Answer from the drawing. Dimensions are ordinates in mm from the lowest x, y and z of the part. A direction names the side the tool comes from. Give positions to 0.01 mm unless a question says otherwise; leave off trailing zeros. Loops run counter-clockwise (first coordinate to the right, second up) from the corner with the lowest first, then second, coordinate; pieces in that order, holes last. Notation, with made-up numbers: (-32, 82) - (-27, 82) arc R26 cw to (-27, 103) - close; hole circle Ø11 at (36.5, 26). An arc over 180 degrees is marked (long way). One line per question, with ' | ' between items. Start each with the question number.
1. Section C-C (x = 27) is taken. Determine the outline of the cut face in (y, z).
2. Section A-A (z = 6.5) is taken. Determine the outline of the cut face in (x, y), plus the area to 3 significant figures.
3. Section B-B (y = 6.25) is taken. Determine the outline of the cut face in (x, z), plus the area to 3 significant figures.
4. For a pull along X with two mould halves and no side action, classify the marked faces 3, 4 and 5 as released by +X, released by -X, zero draft, split by the parting line, or undercut.
5. This flat-tipped pin is pushed along its axis until it touches: pin 1 (12 mm diameter, centred on x = 43.5, y = 10, fed in from -Z). Where does it stop, or does it pass through?
6. Find the intervals of material crossed by line 1 (Y direction, x = 56.5, z = 15); line 2 (X direction, y = 12.25, z = 3.75); line 3 (X direction, y = 1.75, z = 13.75), in increasing order.
7. Section D-D (x = 48.5) is taken. Determine the outline of the cut face in (y, z), plus the area to 3 significant figures.
8. Which of the six approach directions +Z, -Z, +X, -X, +Y, -Y give full straight-line access (tool end or side, diameter ignored) to the marked faces 1 and 2?
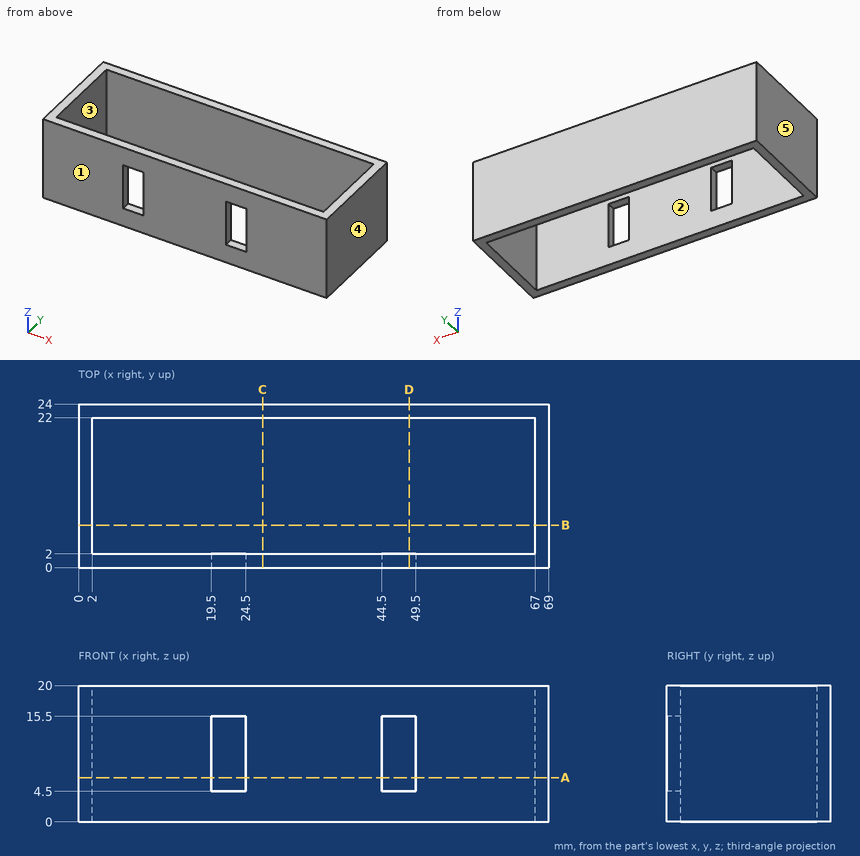
Conclusion:
1) outline: (0, 0) - (2, 0) - (2, 20) - (0, 20) - close; (22, 0) - (24, 0) - (24, 20) - (22, 20) - close
2) outline: (0, 0) - (19.5, 0) - (19.5, 2) - (2, 2) - (2, 22) - (67, 22) - (67, 2) - (49.5, 2) - (49.5, 0) - (69, 0) - (69, 24) - (0, 24) - close; (24.5, 0) - (44.5, 0) - (44.5, 2) - (24.5, 2) - close | area: 336 mm²
3) outline: (0, 0) - (2, 0) - (2, 20) - (0, 20) - close; (67, 0) - (69, 0) - (69, 20) - (67, 20) - close | area: 80.0 mm²
4) face 3: undercut | face 4: released by +X | face 5: released by -X
5) pin 1: through
6) line 1: 0 to 2, 22 to 24 | line 2: 0 to 2, 67 to 69 | line 3: 0 to 19.5, 24.5 to 44.5, 49.5 to 69
7) outline: (0, 0) - (2, 0) - (2, 4.5) - (0, 4.5) - close; (0, 15.5) - (2, 15.5) - (2, 20) - (0, 20) - close; (22, 0) - (24, 0) - (24, 20) - (22, 20) - close | area: 58.0 mm²
8) face 1: +Z, -Z, +X, -X, -Y | face 2: +Z, -Z
